For this review, use the dimensioned drawing (mm, ordinates from the lowest corner) and the shaded views. A direction names the side the tool comes from. Round coordinates to 2 decimals unless told otherwise and drop trailing zeros. Write each loop counter-clockwise with the first axis right and the second up, starting at its lowest first coordinate (ties: lowest second). Pieces come first, ordered by that corner, then holes.
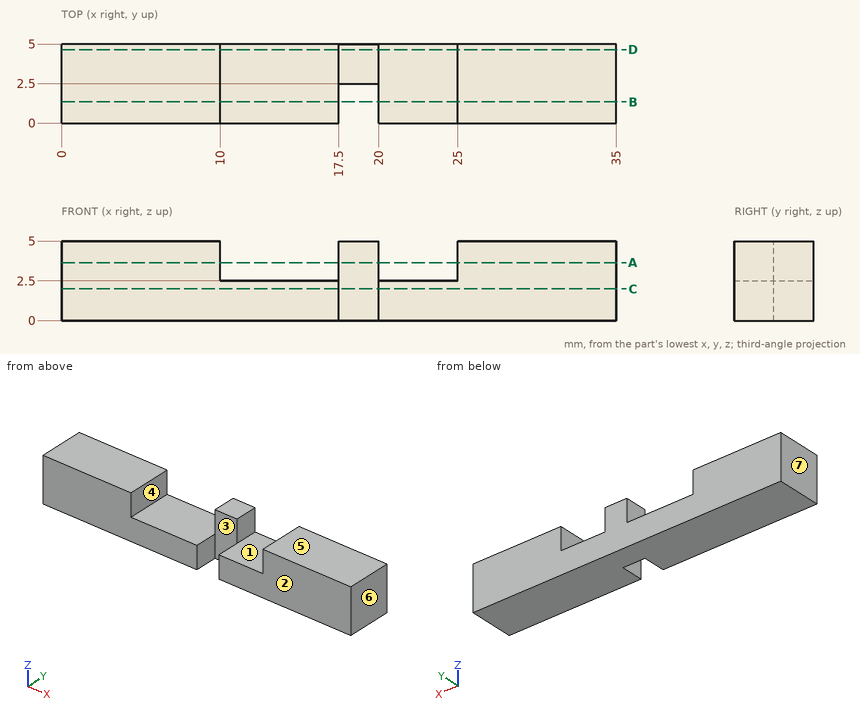
(1) We need section A-A, the plane z = 3.65. Give the boundary of the cut face in (x, y), and give its area (3 significant figures).
Geometry check:
outline: (0, 0) - (10, 0) - (10, 5) - (0, 5) - close; (17.5, 2.5) - (20, 2.5) - (20, 5) - (17.5, 5) - close; (25, 0) - (35, 0) - (35, 5) - (25, 5) - close
area: 106 mm2
(2) For the marked faces 1, 2 and 3, list the 3-axis set-ups (+Z, -Z, +X, -X, +Y, -Y) from which the entire face can be reached by the end or side of a thin tool; tool diameter is ignored.
Geometry check:
face 1: +Z, +Y, -Y
face 2: +Z, -Z, +X, -X, -Y
face 3: +Z, -Z, -Y
(3) We need section C-C, the plane z = 2. Give the boundary of the cut face in (x, y), and give its area (3 significant figures).
Geometry check:
outline: (0, 0) - (17.5, 0) - (17.5, 2.5) - (20, 2.5) - (20, 0) - (35, 0) - (35, 5) - (0, 5) - close
area: 169 mm2
(4) We need section D-D, the plane y = 4.65. Give the boundary of the cut face in (x, z).
Geometry check:
outline: (0, 0) - (35, 0) - (35, 5) - (25, 5) - (25, 2.5) - (20, 2.5) - (20, 5) - (17.5, 5) - (17.5, 2.5) - (10, 2.5) - (10, 5) - (0, 5) - close
(5) We need section B-B, the plane y = 1.35. Give the boundary of the cut face in (x, z), and give its area (3 significant figures).
Geometry check:
outline: (0, 0) - (17.5, 0) - (17.5, 2.5) - (10, 2.5) - (10, 5) - (0, 5) - close; (20, 0) - (35, 0) - (35, 5) - (25, 5) - (25, 2.5) - (20, 2.5) - close
area: 131 mm2
(6) For pin 1 Ø2.5 at (x, y) = (22.5, 1.5) entering from +Z, flat-tipped, find the tip position at first contact; note if it passes through.
Geometry check:
pin 1: stops at z = 2.5
(7) For line 1 along X through (y, z) = (3.05, 3.95); line 2 along X through (y, z) = (1.05, 1.1); line 3 along X through (y, z) = (0.8, 4.75), list the stretches that pass through material, from the lowest coordinate up.
Geometry check:
line 1: x = 0 to 10, 17.5 to 20, 25 to 35
line 2: x = 0 to 17.5, 20 to 35
line 3: x = 0 to 10, 25 to 35
(8) Mouldability with a two-part tool opening along X and no side actions: class the marked faces 4, 5, 6 and 7 as pulls with the +X half, pulls with the -X half, needs draft (parallel to the pull), parting line crosses it, or undercut.
Geometry check:
face 4: undercut
face 5: needs draft
face 6: pulls with the +X half
face 7: pulls with the -X half
